Here's how the part is built. I have some questions about the finished solid (model axes, mm). Round coordinates to 2 decimals unless told otherwise and drop trailing zeros. Order: outer loops, then holes, each group sorted by start corner. A loop starts at its lowest first (then second) coordinate and runs counter-clockwise, first axis right, second up. Notation, with made-up numbers: (28, 22.25) - (78, 22.25) arc R36 cw to (78, 58.25) - close; hole circle Ø7 at (63.25, -7.5). An arc over 180 degrees is marked (long way). One line per item, written item: value.
from build123d import *

# Parameters (mm, degrees)
BASPROSKE_W        = 5
BASPROSKE_H        = 6
TOOTHCUT_DEPTH     = 10.848857802
TEETHCUTS_COUNT    = 10
TEETHCUTS_ANGLE    = 324
BORSKE_R           = 0.4
BORE_DEPTH         = 50.0000508
SKETCH1_R          = 2.35
CUT_EXTRUDE1_DEPTH = 10.693816982


with BuildPart() as part:
    # BasProSke → Base-Revolve (revolve)
    with BuildSketch(Plane(origin=(0, 0, 0), x_dir=(1, 0, 0), z_dir=(0, 1, 0)), mode=Mode.PRIVATE) as base_revolve_sk:
        with Locations((2.5, 3)):
            Rectangle(BASPROSKE_W, BASPROSKE_H)
    revolve(base_revolve_sk.sketch.rotate(Axis((-10, 0, 0), (1, 0, 0)), 180), axis=Axis((-10, 0, 0), (1, 0, 0)))

    # TooCutSke → ToothCut (cut, through all)
    with BuildSketch(Plane(origin=(0, 0, 0), x_dir=(0, 0, -1), z_dir=(1, 0, 0))):
        with BuildLine():
            ThreePointArc((0.59278292, 3.701838653), (0, 3.749), (-0.59278292, 3.701838653))
            ThreePointArc((-0.59278292, 3.701838653), (-0.846593509, 4.924114224), (-1.775771316, 5.757784417))
            ThreePointArc((-1.775771316, 5.757784417), (0, 6.0254), (1.775771316, 5.757784417))
            ThreePointArc((1.775771316, 5.757784417), (0.846593509, 4.924114224), (0.59278292, 3.701838653))
        make_face()
    toothcut = extrude(amount=TOOTHCUT_DEPTH, mode=Mode.SUBTRACT)

    # TeethCuts: ToothCut ×10 about axis
    teethcuts_axis = Axis((-10, 0, 0), (1, 0, 0))
    for i in range(1, TEETHCUTS_COUNT):
        add(toothcut.rotate(teethcuts_axis, i * TEETHCUTS_ANGLE / (TEETHCUTS_COUNT - 1)), mode=Mode.SUBTRACT)

    # BorSke → Bore (cut, symmetric)
    with BuildSketch(Plane(origin=(0, 0, 0), x_dir=(0, 0, -1), z_dir=(1, 0, 0))):
        with Locations(Location((0, 0, 0), (0, 0, 180))):
            Circle(BORSKE_R)
    extrude(amount=BORE_DEPTH, both=True, mode=Mode.SUBTRACT)

    # Sketch1 → Cut-Extrude1 (cut, through all)
    with BuildSketch(Plane(origin=(5, 0, 0), x_dir=(0, 0, -1), z_dir=(1, 0, 0))):
        Circle(SKETCH1_R)
    extrude(amount=-CUT_EXTRUDE1_DEPTH, mode=Mode.SUBTRACT)


solid = part.part
Q1. Will these pins go through, and if not, where does the flat tip stop? pin 1 (2 mm diameter, centred on y = 3.5, z = 5, fed in from -X); pin 2 (4 mm diameter, centred on y = 0, z = 0, fed in from +X); pin 3 (1 mm diameter, centred on x = 3.5, y = -2.5, fed in from -Z); pin 4 (1.5 mm diameter, centred on x = 1, y = -4, fed in from -Z).
Results list:
pin 1: x = 0
pin 2: through
pin 3: z = -4.82
pin 4: z = -4.92
Q2. If we section it at A-A, the plane y = 1.5: Please give me the cut outline in (x, z), then the cut area to 3 significant figures.
Results list:
outline: (0, -3.44) - (5, -3.44) - (5, -1.81) - (0, -1.81) - close; (0, 1.81) - (5, 1.81) - (5, 3.44) - (0, 3.44) - close
area: 16.3 mm²
Q3. If we section it at C-C, the plane z = 5.25: Please give me the cut outline in (x, y), then the cut area to 3 significant figures.
Results list:
outline: (0, -0.63) - (5, -0.63) - (5, 0.63) - (0, 0.63) - close
area: 6.26 mm²
Q4. If we section it at D-D, the plane z = 2.5: Please give me the cut outline in (x, y).
Results list:
outline: (0, -2.79) - (5, -2.79) - (5, 2.79) - (0, 2.79) - close
Q5. If we section it at B-B, the plane z = 0: Please give me the cut outline in (x, y), then the cut area to 3 significant figures.
Results list:
outline: (0, -3.75) - (5, -3.75) - (5, -2.35) - (0, -2.35) - close; (0, 2.35) - (5, 2.35) - (5, 3.75) - (0, 3.75) - close
area: 14.0 mm²
Q6. If I drill on line 1 along Y through (x, z) = (1.55, 0); line 2 along Z through (x, y) = (1.85, -0.25); line 3 along Y through (x, z) = (1.1, 1.5), over which ranges is the centre line in solid material (lowest first)?
Results list:
line 1: -3.75 to -2.35, 2.35 to 3.75
line 2: -5.87 to -2.34, 2.34 to 5.87
line 3: -5.61 to -1.81, 1.81 to 5.61
